Source: CAD feature listing. Evaluate the final solid. Frame: model axes, mm. Face numbers are marked on the shaded views. A direction names the side the tool comes from. Round coordinates to 2 decimals unless told otherwise and drop trailing zeros. Write each loop counter-clockwise with the first axis right and the second up, starting at its lowest first coordinate (ties: lowest second). Pieces come first, ordered by that corner, then holes. Notation, with made-up numbers: (1.25, -17.75) -> (8.25, -17.75) arc R13 cw to (8.25, 7.25) -> close; hole circle Ø7 at (51.25, -26). An arc over 180 degrees is marked (long way). Put each result on its own line as item: value.
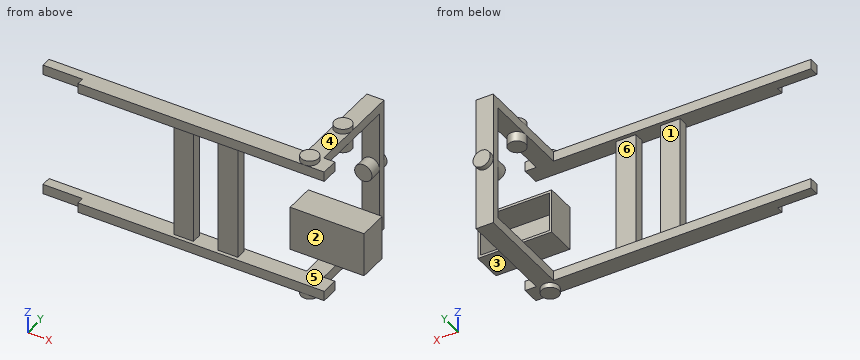
```python
from build123d import *

# Parameters (mm, degrees)
BOSS_EXTRUDE1_DEPTH      = 50.8
BOSS_EXTRUDE2_DEPTH      = 50.8
SKETCH5_W                = 101.6
SKETCH5_H                = 50.8
BOSS_EXTRUDE3_DEPTH      = 596.9
SKETCH6_R                = 44.45
BOSS_EXTRUDE4_DEPTH      = 25.4
SKETCH7_W                = 88.9
SKETCH7_H                = 50.8
BOSS_EXTRUDE5_DEPTH      = 508
SKETCH8_W                = 88.9
SKETCH8_H                = 38.1
BOSS_EXTRUDE6_DEPTH      = 596.9
SKETCH10_W               = 381
SKETCH10_H               = 152.4
BOSS_EXTRUDE7_DEPTH      = 228.6
CUT_EXTRUDE1_DEPTH       = 139.7
BOSS_EXTRUDE8_DEPTH      = 25.4
BOSS_EXTRUDE8_DEPTH_BACK = 101.6
SKETCH13_R               = 44.45
BOSS_EXTRUDE9_DEPTH      = 25.4
BOSS_EXTRUDE9_DEPTH_BACK = 101.6
SKETCH14_R               = 44.45
BOSS_EXTRUDE10_START     = 25.4
SKETCH15_R               = 44.45
BOSS_EXTRUDE10_DEPTH     = 25.4


with BuildPart() as part:
    # Sketch1 → Boss-Extrude1 (new body)
    with BuildSketch(Plane.XY):
        Polygon((0, 0), (1473.2, 0), (1473.2, -88.9), (203.2, -88.9), (203.2, -50.8), (0, -50.8), align=None)
    extrude(amount=-BOSS_EXTRUDE1_DEPTH)



with BuildPart() as body_2:
    # Sketch4 → Boss-Extrude2 (new body)
    with BuildSketch(Plane.XY.offset(596.9)):
        Polygon((0, 0), (1473.2, 0), (1473.2, -88.9), (203.2, -88.9), (203.2, -50.8), (0, -50.8), align=None)
    extrude(amount=BOSS_EXTRUDE2_DEPTH)


with BuildPart() as part_1:
    add(part.part)

    add(body_2.part)  # Boss-Extrude3 merges body 2
    # Sketch5 → Boss-Extrude3 (add)
    with BuildSketch(Plane.XY):
        with Locations((965.2, -44.45)):
            Rectangle(SKETCH5_W, SKETCH5_H)
        with Locations((736.6, -44.45)):
            Rectangle(SKETCH5_W, SKETCH5_H)
    extrude(amount=BOSS_EXTRUDE3_DEPTH)

    # Sketch6 → Boss-Extrude4 (add)
    with BuildSketch(Plane.XY.offset(647.7)):
        with Locations(Location((1371.6, -44.45, 0), (0, 0, 270))):
            Circle(SKETCH6_R)
    extrude(amount=BOSS_EXTRUDE4_DEPTH)

    # Sketch7 → Boss-Extrude5 (add)
    with BuildSketch(Plane(origin=(0, 0, 0), x_dir=(1, 0, 0), z_dir=(0, 1, 0))):
        with Locations((1371.6, -622.3)):
            Rectangle(SKETCH7_W, SKETCH7_H)
        with Locations((1371.6, 25.4)):
            Rectangle(SKETCH7_W, SKETCH7_H)
    extrude(amount=BOSS_EXTRUDE5_DEPTH)

    # Sketch8 → Boss-Extrude6 (add)
    with BuildSketch(Plane.XY):
        with Locations((1371.6, 488.95)):
            Rectangle(SKETCH8_W, SKETCH8_H)
    extrude(amount=BOSS_EXTRUDE6_DEPTH)

    # Sketch10 → Boss-Extrude7 (add)
    with BuildSketch(Plane.XY):
        with Locations((1371.6, 177.8)):
            Rectangle(SKETCH10_W, SKETCH10_H)
    extrude(amount=BOSS_EXTRUDE7_DEPTH)

    # Sketch11 → Cut-Extrude1 (cut)
    with BuildSketch(Plane(origin=(0, 254, 0), x_dir=(1, 0, 0), z_dir=(0, 1, 0))):
        Polygon((1549.4, -12.7), (1416.05, -12.7), (1327.15, -12.7), (1193.8, -12.7), (1193.8, -215.9), (1549.4, -215.9), align=None)
    extrude(amount=-CUT_EXTRUDE1_DEPTH, mode=Mode.SUBTRACT)

    # Sketch13 → Boss-Extrude8 (add, two sides: drawn at the far end of the back side and taken through both)
    with BuildSketch(Plane(origin=(0, 508, 0), x_dir=(1, 0, 0), z_dir=(0, 1, 0)).offset(-BOSS_EXTRUDE8_DEPTH_BACK)):
        with Locations(Location((1371.6, -298.45, 0), (0, 0, 270))):
            Circle(SKETCH13_R)
    extrude(amount=BOSS_EXTRUDE8_DEPTH + BOSS_EXTRUDE8_DEPTH_BACK)

    # Sketch14 → Boss-Extrude9 (add, two sides: drawn at the far end of the back side and taken through both)
    with BuildSketch(Plane.XY.offset(647.7).offset(-BOSS_EXTRUDE9_DEPTH_BACK)):
        with Locations((1371.6, 234.95)):
            Circle(SKETCH14_R)
    extrude(amount=BOSS_EXTRUDE9_DEPTH + BOSS_EXTRUDE9_DEPTH_BACK)

    # Sketch15 → Boss-Extrude10 (add)
    with BuildSketch(Plane(origin=(0, 0, -50.8), x_dir=(-1, 0, 0), z_dir=(0, 0, -1)).offset(BOSS_EXTRUDE10_START)):
        with Locations(Location((-1371.6, -44.45, 0), (0, 0, 270))):
            Circle(SKETCH15_R)
    extrude(amount=-BOSS_EXTRUDE10_DEPTH)


solid = part_1.part
```
Q1. Reachability of the marked faces 1, 2 and 3 from +Z, -Z, +X, -X, +Y, -Y: full face, straight path, thin tool, end or side. Return the list, or none.
Ans:
face 1: +X, -X, +Y
face 2: +X, -X, -Y
face 3: -Z, +X, +Y
Q2. Material intervals for line 1 (Y direction, x = 1393.5, z = 36); line 2 (X direction, y = 505, z = 28.5); line 3 (Z direction, x = 607, y = -55.5), sorted ascending. Write a range as [from, to].
Ans:
line 1: y = [101.6, 114.3], [469.9, 508]
line 2: x = [1327.15, 1416.05]
line 3: z = [-50.8, 0], [596.9, 647.7]
Q3. Pin query (flat end, axial travel): pin 1 (10 mm diameter, centred on x = 1357, z = 364.5, fed in from -Y); pin 2 (15 mm diameter, centred on x = 712.5, z = -35.5, fed in from +Y); pin 3 (3 mm diameter, centred on x = 402.5, y = -2.5, fed in from -Z). Return the tip coordinate at first contact, or that it passes through.
Ans:
pin 1: stops at y = 469.9
pin 2: stops at y = 0
pin 3: stops at z = -50.8
Q4. Cut plane C-C on z = 113. Output: boundary loops of the cut face in (x, y).
Ans:
outline: (685.8, -69.85) -> (787.4, -69.85) -> (787.4, -19.05) -> (685.8, -19.05) -> close; (914.4, -69.85) -> (1016, -69.85) -> (1016, -19.05) -> (914.4, -19.05) -> close; (1181.1, 101.6) -> (1562.1, 101.6) -> (1562.1, 254) -> (1549.4, 254) -> (1549.4, 114.3) -> (1193.8, 114.3) -> (1193.8, 254) -> (1181.1, 254) -> close; (1327.15, 469.9) -> (1416.05, 469.9) -> (1416.05, 508) -> (1327.15, 508) -> close
Q5. Cut plane A-A on y = 424. Output: boundary loops of the cut face in (x, z).
Ans:
outline: (1327.15, -50.8) -> (1416.05, -50.8) -> (1416.05, 0) -> (1327.15, 0) -> close; circle Ø88.9 at (1371.6, 298.45); (1327.15, 596.9) -> (1416.05, 596.9) -> (1416.05, 647.7) -> (1327.15, 647.7) -> close
Q6. Cut plane D-D on x = 1238.5. Output: boundary loops of the cut face in (y, z).
Ans:
outline: (-88.9, -50.8) -> (0, -50.8) -> (0, 0) -> (-88.9, 0) -> close; (-88.9, 596.9) -> (0, 596.9) -> (0, 647.7) -> (-88.9, 647.7) -> close; (101.6, 0) -> (254, 0) -> (254, 12.7) -> (114.3, 12.7) -> (114.3, 215.9) -> (254, 215.9) -> (254, 228.6) -> (101.6, 228.6) -> close
Q7. Draft query along Y for the marked faces 4, 5 and 6. Return one class per face: +Y half, -Y half, draft (parallel to the pull), parting line (faces both ways), or undercut.
Ans:
face 4: undercut
face 5: draft
face 6: +Y half
Q8. Cut plane B-B on x = 269. Output: boundary loops of the cut face in (y, z), and give its area (3 significant figures).
Ans:
outline: (-88.9, -50.8) -> (0, -50.8) -> (0, 0) -> (-88.9, 0) -> close; (-88.9, 596.9) -> (0, 596.9) -> (0, 647.7) -> (-88.9, 647.7) -> close
area: 9,030 mm^2
